Here's how the part is built. I have some questions about the finished solid (model axes, mm). Coordinates: 2 decimals unless noted, no trailing zeros. Loops run counter-clockwise (first coordinate to the right, second up) from the corner with the lowest first, then second, coordinate; pieces in that order, holes last. Notation, with made-up numbers: (11.5, 56) -> (55.5, 56) arc R26 cw to (55.5, 92) -> close; hole circle Ø8 at (30, 65). An arc over 180 degrees is marked (long way). Answer as a JSON object with one key per item and string values. Group by question number.
Q1. Thinking about a two-plate mould opening in Z: for faces 1 (the cylindrical face through (159.13, -0.04, -5.74)), 2 (the cylindrical face through (79.599, 0.035, 252.763)), 3 (the flat face through (4, 2.5, -4)), which applies, released by +Z, released by -Z, zero draft, split by the parting line, or undercut?
Q2. I want a section at C-C on y = 0.85. Count the separate pieces of the cut face and the enclosed holes in it, then the cut area to 3 significant figures.
Q3. I want a section at A-A on z = 185. Write out the boundary of the cut face in (x, y), then the cut area to 3 significant figures.
Q4. I want a section at B-B on x = 185. Write out the boundary of the cut face in (y, z), then the cut area to 3 significant figures.
Q5. I'm going to push flat-ended pins straight in: pin 1 (4 mm diameter, centred on x = -160.95, z = 24.05, fed in from +Y); pin 2 (2 mm diameter, centred on y = -1, z = 99.5, fed in from -X). Where does each tip first touch, or does it pass through?
Q6. I want a section at D-D on z = -75. Write out the boundary of the cut face in (x, y).
Q7. I need wall thicknesses on line 1 (X direction, y = 1.5, z = 0); line 2 (Z direction, x = -209.05, y = 0.95); line 3 (X direction, y = 0.1, z = -185). Which ranges of each line are inside material? Lowest first, please.
```python
from build123d import *

# Parameters (mm, degrees)
SKETCH1_R           = 265
SKETCH1_R_2         = 26.5
SKETCH1_R_3         = 2.3
SKETCH1_R_4         = 9.1
SKETCH1_R_5         = 6
BOSS_EXTRUDE1_DEPTH = 2.5


with BuildPart() as part:
    # Sketch1 → Boss-Extrude1 (new, symmetric)
    with BuildSketch(Plane(origin=(0, 0, 0), x_dir=(1, 0, 0), z_dir=(0, 1, 0))):
        with Locations(Location((0, 0, 0), (0, 0, 270))):
            Circle(SKETCH1_R)
        with Locations(Location((-185, 0, 0), (0, 0, 270))):
            Circle(SKETCH1_R_2, mode=Mode.SUBTRACT)
        with Locations(Location((185, 0, 0), (0, 0, 270))):
            Circle(SKETCH1_R_2, mode=Mode.SUBTRACT)
        with Locations(Location((-209.05, 24.05, 0), (0, 0, 270))):
            Circle(SKETCH1_R_3, mode=Mode.SUBTRACT)
        with Locations(Location((-160.95, 24.05, 0), (0, 0, 270))):
            Circle(SKETCH1_R_3, mode=Mode.SUBTRACT)
        with Locations(Location((-160.95, -24.05, 0), (0, 0, 270))):
            Circle(SKETCH1_R_3, mode=Mode.SUBTRACT)
        with Locations(Location((-209.05, -24.05, 0), (0, 0, 270))):
            Circle(SKETCH1_R_3, mode=Mode.SUBTRACT)
        with Locations(Location((209.05, -24.05, 0), (0, 0, 270))):
            Circle(SKETCH1_R_3, mode=Mode.SUBTRACT)
        with Locations(Location((160.95, -24.05, 0), (0, 0, 270))):
            Circle(SKETCH1_R_3, mode=Mode.SUBTRACT)
        with Locations(Location((160.95, 24.05, 0), (0, 0, 270))):
            Circle(SKETCH1_R_3, mode=Mode.SUBTRACT)
        with Locations(Location((209.05, 24.05, 0), (0, 0, 270))):
            Circle(SKETCH1_R_3, mode=Mode.SUBTRACT)
        with Locations(Location((0, 185, 0), (0, 0, 270))):
            Circle(SKETCH1_R_4, mode=Mode.SUBTRACT)
        with Locations(Location((-130.81475452, -130.81475452, 0), (0, 0, 270))):
            Circle(SKETCH1_R_5, mode=Mode.SUBTRACT)
        with Locations(Location((130.81475452, -130.81475452, 0), (0, 0, 270))):
            Circle(SKETCH1_R_5, mode=Mode.SUBTRACT)
        with Locations(Location((0, -185, 0), (0, 0, 270))):
            Circle(SKETCH1_R_5, mode=Mode.SUBTRACT)
    extrude(amount=BOSS_EXTRUDE1_DEPTH, both=True)


solid = part.part
```
Result set:
{
 "1": {"face 1": "undercut", "face 2": "split by the parting line", "face 3": "zero draft"},
 "2": {"separate pieces": "1", "enclosed holes": "14", "area": "215,000 mm²"},
 "3": {"outline": "(-189.74, -2.5) -> (-6, -2.5) -> (-6, 2.5) -> (-189.74, 2.5) -> close; (6, -2.5) -> (189.74, -2.5) -> (189.74, 2.5) -> (6, 2.5) -> close", "area": "1,840 mm²"},
 "4": {"outline": "(-2.5, -189.74) -> (2.5, -189.74) -> (2.5, -26.5) -> (-2.5, -26.5) -> close; (-2.5, 26.5) -> (2.5, 26.5) -> (2.5, 189.74) -> (-2.5, 189.74) -> close", "area": "1,630 mm²"},
 "5": {"pin 1": "passes through", "pin 2": "stops at x = -246.01"},
 "6": {"outline": "(-254.17, -2.5) -> (254.17, -2.5) -> (254.17, 2.5) -> (-254.17, 2.5) -> close"},
 "7": {"line 1": "x = -265 to -211.5, -158.5 to 158.5, 211.5 to 265", "line 2": "z = -162.86 to -26.35, -21.75 to -11.13, 11.13 to 21.75, 26.35 to 162.86", "line 3": "x = -189.74 to -9.1, 9.1 to 189.74"}
}
